Autodesk Inventor part; units mm, degrees
ref_plane "YZ Plane" through (0, 0, 0) normal (1, 0, 0) x (0, 1, 0)
ref_plane "XZ Plane" through (0, 0, 0) normal (0, 1, 0) x (-1, 0, 0)
ref_plane "XY Plane" through (0, 0, 0) normal (0, 0, 1) x (1, 0, 0)
sketch "Sketch1" plane through (0, 0, 0) normal (1, 0, 0) x (0, 1, 0)
  line L0 (-50, 45) -> (50, 45)
  line L1 (50, 45) -> (50, -45)
  line L2 (50, -45) -> (-50, -45)
  line L3 (-50, -45) -> (-50, 45)
  point P0 (0, 0)
  dimension "d0" = 100
  dimension "d35" = 90
  dimension "d36" = 50
  dimension "d37" = 45
extrude "Plate1" add sketch "Sketch1" along normal blind 3
sketch "Sketch2" plane through (-3, 53, -45) normal (0, 1, 0) x (-1, 0, 0)
  line L0 (0, 90) -> (0, 0)
  line L1 (0, 0) -> (19, 0)
  line L2 (19, 0) -> (19, 90)
  line L3 (19, 90) -> (0, 90)
edge flange "Flange1" height 25 angle 90 thickness 3 bend radius 3 thickness toward (0, 1, 0) relief tear relief width 3 relief depth 1.5 corner gap 3 corner form 0 edges at (0, 50, 0) (0, -50, 0) wall of the first edge with corners at (-3, 53, 45) (-3, 53, -45) (-22, 53, -45) (-22, 53, 45)
bend "Bend1"
corner "Corner1"
sketch "Sketch3" plane through (6, -50, 48) normal (0, 0, 1) x (1, 0, 0)
  line L0 (0, 100) -> (0, 0)
  line L1 (0, 0) -> (23.4696, 0)
  line L2 (23.4696, 0) -> (23.4696, 100)
  line L3 (23.4696, 100) -> (0, 100)
edge flange "Flange2" height 29.4696 angle 90 thickness 3 bend radius 3 thickness toward (0, 0, 1) relief tear relief width 3 relief depth 1.5 corner gap 3 corner form 0 edges at (3, 0, 45) (3, 0, -45) wall of the first edge with corners at (6, 50, 48) (6, -50, 48) (29.4696, -50, 48) (29.4696, 50, 48)
bend "Bend2"
corner "Corner2"
sketch "Sketch4" plane through (3, 0, 0) normal (1, 0, 0) x (0, 0, -1)
  line L0 (-45, 50) -> (45, 50)
  line L1 (-45, -50) -> (-45, 50)
  line L2 (45, -50) -> (-45, -50)
  line L3 (45, 50) -> (45, -50)
  circle A0 centre (-31.5962, 12.4637) radius 7.62 construction
  circle A1 centre (1.5, 12.4637) radius 12.7 construction
  circle A2 centre (34.5962, 12.4637) radius 7.62 construction
  circle A3 centre (1.5, -25.7125) radius 25.4 construction
  circle A4 centre (1.5, 12.4637) radius 25.4 construction
  line L4 (26.9762, 12.4637) -> (26.9, 12.4637) construction
  line L5 (-23.9762, 12.4637) -> (-23.9, 12.4637) construction
  line L6 (1.5, -0.3125) -> (1.5, -0.2363) construction
  line L7 (-33.5, -12.8649) -> (-29.6924, 37.7923) construction
  line L8 (36.5, -12.8649) -> (32.6924, 37.7923) construction
  point P0 (0, 0)
  dimension "d24" = 25.4
  dimension "d25" = 15.24
  dimension "d27" = 50.8
  dimension "d23" = 0.0762
  dimension "d26" = 50.8
  dimension "d34" = 66.1924
  dimension "d38" = 24.2875
  dimension "d40" = 46.5
  dimension "d41" = 43.5
  dimension "d42" = 50.8
  dimension "d45" = 70
sketch "Sketch5" plane through (3, 0, 0) normal (1, 0, 0) x (0, 0, -1)
  circle A0 centre (-31.5962, 12.4637) radius 9.525
  circle A1 centre (34.5962, 12.4637) radius 9.525
  circle A2 centre (1.5, 12.4637) radius 11.1125
  circle A3 centre (1.5, -25.7125) radius 14.2875
  line L0 (-33.5, -12.8649) -> (-29.6924, 37.7923) construction
  line L1 (36.5, -12.8649) -> (32.6924, 37.7923) construction
  circle A4 centre (-29.6924, 37.7923) radius 3
  circle A5 centre (32.6924, 37.7923) radius 3
  circle A6 centre (36.5, -12.8649) radius 3
  circle A7 centre (-33.5, -12.8649) radius 3
  point P0 (0, 0)
  dimension "d28" = 19.05
  dimension "d30" = 22.225
  dimension "d31" = 28.575
  dimension "d44" = 6
extrude "Cut1" cut sketch "Sketch5" against normal blind 3
sketch "Sketch7" plane through (29.4696, -50, 51) normal (0, 0, 1) x (1, 0, 0)
  line L0 (-23.4696, 100) -> (-23.4696, 0)
  line L1 (0, 100) -> (0, 0)
  line L2 (-23.4696, 100) -> (0, 100)
  circle A0 centre (-11.7348, 90) radius 3
  circle A1 centre (-11.7348, 55) radius 3
  circle A2 centre (-11.7348, 20) radius 3
  point P0 (-29.4696, 50)
  dimension "d72" = 6
  dimension "d74" = 11.7348
  dimension "d75" = 11.7348
  dimension "d76" = 10
  dimension "d79" = 35
extrude "Cut3" cut sketch "Sketch7" against normal through all
sketch "Sketch8" plane through (-22, 56, 45) normal (0, 1, 0) x (1, 0, 0)
  line L0 (19, 0) -> (19, 90)
  line L1 (0, 0) -> (0, 90)
  line L2 (19, 0) -> (0, 0)
  circle A0 centre (9.5, 15) radius 3
  circle A1 centre (9.5, 35) radius 3
  circle A2 centre (9.5, 55) radius 3
  circle A3 centre (9.5, 75) radius 3
  point P0 (22, 45)
  dimension "d86" = 6
  dimension "d88" = 9.5
  dimension "d89" = 9.5
  dimension "d90" = 15
  dimension "d93" = 20
extrude "Cut4" cut sketch "Sketch8" against normal through all
sketch "Sketch9" plane through (0, 0, 0) normal (-1, 0, 0) x (0, 0, 1)
  circle A0 centre (-1.5, 12.4637) radius 11.1125
  circle A1 centre (-32.6924, 37.7923) radius 3
  circle A2 centre (-34.5962, 12.4637) radius 9.525
  line L0 (45, 50) -> (-45, 50)
  arc A3 (-20.715, 19.4163) -> (-27.9683, 26.5028) centre (-34.5962, 12.4637) ccw
  arc A4 (-28.1286, 30.0352) -> (-24.3769, 41.235) centre (-32.6924, 37.7923) ccw
  arc A5 (-5.9768, 28.9802) -> (-17.1032, 19.4907) centre (-1.5, 12.4637) ccw
  line L1 (-6.5, 44) -> (-22.529, 44)
  arc A6 (-28.1286, 30.0352) -> (-27.9683, 26.5028) centre (-27.1145, 28.3114) ccw
  arc A7 (-22.529, 44) -> (-24.3769, 41.235) centre (-22.529, 42) ccw
  arc A8 (-20.715, 19.4163) -> (-17.1032, 19.4907) centre (-18.9268, 20.3119) ccw
  circle A9 centre (-36.5, -12.8649) radius 3
  circle A10 centre (-1.5, -25.7125) radius 14.2875
  line L2 (-45, 50) -> (-45, -50)
  line L3 (-45, -50) -> (45, -50)
  line L4 (-4.5, 30.9106) -> (-4.5, 42)
  arc A11 (-4.5, 42) -> (-6.5, 44) centre (-6.5, 42) ccw
  arc A12 (-5.9768, 28.9802) -> (-4.5, 30.9106) centre (-6.5, 30.9106) ccw
  line L5 (-1.5, 12.4637) -> (-1.5, -25.7125)
  arc A13 (-21.6278, -23.1723) -> (-15.3483, -40.5384) centre (-1.5, -25.7125) ccw
  arc A14 (-36.9091, -21.8555) -> (-30.3842, -19.4676) centre (-36.5, -12.8649) ccw
  line L6 (-39, -23.8535) -> (-39, -42)
  line L7 (-16.7135, -44) -> (-37, -44)
  arc A15 (-39, -42) -> (-37, -44) centre (-37, -42) ccw
  arc A16 (-16.7135, -44) -> (-15.3483, -40.5384) centre (-16.7135, -42) ccw
  arc A17 (-36.9091, -21.8555) -> (-39, -23.8535) centre (-37, -23.8535) ccw
  line L8 (-28.3359, -19.0574) -> (-22.9229, -21.0444)
  arc A18 (-28.3359, -19.0574) -> (-30.3842, -19.4676) centre (-29.0251, -20.9349) ccw
  arc A19 (-21.6278, -23.1723) -> (-22.9229, -21.0444) centre (-23.6121, -22.9219) ccw
  arc A20 (-27.5648, -11.7869) -> (-30.828, -5.8772) centre (-36.5, -12.8649) ccw
  arc A21 (-8.7645, -6.7702) -> (-18.4911, -14.6272) centre (-1.5, -25.7125) ccw
  arc A22 (-17.1032, 5.4367) -> (-8.6455, -3.0855) centre (-1.5, 12.4637) ccw
  arc A23 (-30.1414, -2.4084) -> (-20.715, 5.5111) centre (-34.5962, 12.4637) ccw
  line L9 (-26.2684, -13.4249) -> (-20.8554, -15.4119)
  arc A24 (-27.5648, -11.7869) -> (-26.2684, -13.4249) centre (-25.5792, -11.5474) ccw
  arc A25 (-30.1414, -2.4084) -> (-30.828, -5.8772) centre (-29.5675, -4.3243) ccw
  arc A26 (-17.1032, 5.4367) -> (-20.715, 5.5111) centre (-18.9268, 4.6155) ccw
  arc A27 (-8.7645, -6.7702) -> (-8.6455, -3.0855) centre (-9.4807, -4.9028) ccw
  arc A28 (-20.8554, -15.4119) -> (-18.4911, -14.6272) centre (-20.1662, -13.5344) ccw
  arc A29 (24.9683, 26.5028) -> (17.715, 19.4163) centre (31.5962, 12.4637) ccw
  arc A30 (21.3769, 41.235) -> (25.1286, 30.0352) centre (29.6924, 37.7923) ccw
  arc A31 (14.1032, 19.4907) -> (2.9768, 28.9802) centre (-1.5, 12.4637) ccw
  line L10 (3.5, 44) -> (19.529, 44)
  arc A32 (24.9683, 26.5028) -> (25.1286, 30.0352) centre (24.1145, 28.3114) ccw
  arc A33 (21.3769, 41.235) -> (19.529, 44) centre (19.529, 42) ccw
  arc A34 (14.1032, 19.4907) -> (17.715, 19.4163) centre (15.9268, 20.3119) ccw
  line L11 (1.5, 30.9106) -> (1.5, 42)
  arc A35 (3.5, 44) -> (1.5, 42) centre (3.5, 42) ccw
  arc A36 (1.5, 30.9106) -> (2.9768, 28.9802) centre (3.5, 30.9106) ccw
  arc A37 (12.3483, -40.5384) -> (18.6278, -23.1723) centre (-1.5, -25.7125) ccw
  arc A38 (27.3842, -19.4676) -> (33.9091, -21.8555) centre (33.5, -12.8649) ccw
  line L12 (36, -23.8535) -> (36, -42)
  line L13 (13.7135, -44) -> (34, -44)
  arc A39 (34, -44) -> (36, -42) centre (34, -42) ccw
  arc A40 (12.3483, -40.5384) -> (13.7135, -44) centre (13.7135, -42) ccw
  arc A41 (36, -23.8535) -> (33.9091, -21.8555) centre (34, -23.8535) ccw
  line L14 (25.3359, -19.0574) -> (19.9229, -21.0444)
  arc A42 (27.3842, -19.4676) -> (25.3359, -19.0574) centre (26.0251, -20.9349) ccw
  arc A43 (19.9229, -21.0444) -> (18.6278, -23.1723) centre (20.6121, -22.9219) ccw
  arc A44 (27.828, -5.8772) -> (24.5648, -11.7869) centre (33.5, -12.8649) ccw
  arc A45 (15.4911, -14.6272) -> (5.7645, -6.7702) centre (-1.5, -25.7125) ccw
  arc A46 (5.6455, -3.0855) -> (14.1032, 5.4367) centre (-1.5, 12.4637) ccw
  arc A47 (17.715, 5.5111) -> (27.1414, -2.4084) centre (31.5962, 12.4637) ccw
  line L15 (23.2684, -13.4249) -> (17.8554, -15.4119)
  arc A48 (23.2684, -13.4249) -> (24.5648, -11.7869) centre (22.5792, -11.5474) ccw
  arc A49 (27.828, -5.8772) -> (27.1414, -2.4084) centre (26.5675, -4.3243) ccw
  arc A50 (17.715, 5.5111) -> (14.1032, 5.4367) centre (15.9268, 4.6155) ccw
  arc A51 (5.6455, -3.0855) -> (5.7645, -6.7702) centre (6.4807, -4.9028) ccw
  arc A52 (15.4911, -14.6272) -> (17.8554, -15.4119) centre (17.1662, -13.5344) ccw
  point P0 (0, 0)
  point P1 (-26.176, 44)
  dimension "d100" = 6
  dimension "d101" = 6
  dimension "d102" = 6
  dimension "d103" = 6
  dimension "d105" = 2
  dimension "d108" = 6
  dimension "d109" = 6
  dimension "d110" = 3
  dimension "d111" = 6
  dimension "d112" = 6
  dimension "d113" = 3
  dimension "d114" = 6
cut "Cut5" [suppressed]
equation "\"d32\" = Thickness"
equation "\"d3\" = BendReliefWidth"
equation "\"d4\" = BendReliefDepth"
equation "\"d5\" = MinimumRemnant"
equation "\"d6\" = BendRadius"
equation "\"d9\" = BendRadius"
equation "\"d10\" = CornerReliefSize"
equation "\"d11\" = GapSize"
equation "\"d12\" = JacobiRadiusSize"
equation "\"d13\" = BendReliefWidth"
equation "\"d14\" = BendReliefDepth"
equation "\"d15\" = MinimumRemnant"
equation "\"d16\" = BendRadius"
equation "\"d19\" = BendRadius"
equation "\"d20\" = CornerReliefSize"
equation "\"d21\" = GapSize"
equation "\"d22\" = JacobiRadiusSize"
equation "\"BendRadius\" = Thickness"
equation "\"BendReliefWidth\" = Thickness"
equation "\"BendReliefDepth\" = 0.5 * Thickness"
equation "\"CornerReliefSize\" = 4 * Thickness"
equation "\"MinimumRemnant\" = 2 * Thickness"
equation "\"TransitionRadius\" = BendRadius"
equation "\"JacobiRadiusSize\" = BendRadius"
equation "\"GapSize\" = Thickness"
equation "\"d2\" = BendRadius"
properties part number "GearboxPlate" material "Aluminum 6061"
Part model, mm, in its own coordinate system. A direction names the side the tool comes from. Round coordinates to 2 decimals unless told otherwise and drop trailing zeros. Write each loop counter-clockwise with the first axis right and the second up, starting at its lowest first coordinate (ties: lowest second). Pieces come first, ordered by that corner, then holes. Notation, with made-up numbers: (3, 85.25) -> (8, 85.25) arc R27 cw to (8, 113.25) -> close; hole circle Ø7 at (64, 50). An arc over 180 degrees is marked (long way). Return JSON: item names as keys, results as strings. Group by question number.
Q1. Probe L1, parallel to Y at x = -14.5, z = 15.5; L2, parallel to Y at x = 1, z = -36; L3, parallel to Z at x = 19, y = -1. List the from-to ranges inside material, lowest first. Write a range as [from, to].
Q2. Which spindle directions (+Z, -Z, +X, -X, +Y, -Y) get a long thin tool onto all of the face, cutting with end or side? Do faces 1 (the flat face through (-10, 54, 45)), 2 (the flat face through (18, 1, -48)), 3 (the cylindrical face through (-0.9, -52.14, 0.63)). Say none if no direction does.
Q3. Saw through at D-D on x = 7.5. Write the cut outline in (y, z).
Q4. Saw through at B-B on z = -1.5. Write the cut outline in (x, y) (3 decimals), plus the area to 3 significant figures.
Q5. Pin check, flat tips, straight feed: pin 1 (6 mm diameter, centred on x = -4.5, y = -19, fed in from -Z); pin 2 (2 mm diameter, centred on y = -37.5, z = -11, fed in from +X); pin 3 (3 mm diameter, centred on y = -2, z = -7, fed in from -X); pin 4 (5 mm diameter, centred on x = 0, y = 22, fed in from +Z). Stop position of each tip, or through.
Q6. Saw through at C-C on y = 18. Write the cut outline in (x, z), plus the area to 3 significant figures.
Q7. Saw through at A-A on x = -7.5. Write the cut outline in (y, z), plus the area to 3 significant figures.
Q8. Mould opens along X. For faces 4 (the flat face through (0, -1, 1)), 5 (the flat face through (15, -50, -49)), 6 (the cylindrical face through (-14.71, -54.48, -32.03)), 7 (the cylindrical face through (-14.71, -54.48, 7.97)) say: pulls with the +X half, pulls with the -X half, needs draft (parallel to the pull), parting line crosses it, or undercut.
Answer:
{
 "1": {"L1": "[-56, -53], [53, 56]", "L2": "[-54.47, -15.82], [-9.91, 3.04], [21.88, 54.47]", "L3": "[-51, -48], [48, 51]"},
 "2": {"face 1": "+Z, +X, -X, +Y", "face 2": "+X, +Y, -Y", "face 3": "+Z, -Z, -X"},
 "3": {"outline": "(-50, -51) -> (50, -51) -> (50, -48) -> (-50, -48) -> close; (-50, 48) -> (50, 48) -> (50, 51) -> (-50, 51) -> close"},
 "4": {"outline": "(-22, -56) -> (-3, -56) arc R6 ccw to (3, -50) -> (3, -40) -> (0, -40) -> (0, -50) arc R3 cw to (-3, -53) -> (-22, -53) -> close; (-22, 53) -> (-3, 53) arc R3 cw to (0, 50) -> (0, 23.576) -> (3, 23.576) -> (3, 50) arc R6 ccw to (-3, 56) -> (-22, 56) -> close; (0, -11.425) -> (3, -11.425) -> (3, 1.351) -> (0, 1.351) -> close", "area": "304 mm2"},
 "5": {"pin 1": "through", "pin 2": "x = 3", "pin 3": "x = 0", "pin 4": "z = 49.87"},
 "6": {"outline": "(0, -45) arc R6 ccw to (6, -51) -> (29.47, -51) -> (29.47, -48) -> (6, -48) arc R3 cw to (3, -45) -> (3, -42.35) -> (0, -42.35) -> close; (0, -26.85) -> (3, -26.85) -> (3, -11.14) -> (0, -11.14) -> close; (0, 8.14) -> (3, 8.14) -> (3, 23.85) -> (0, 23.85) -> close; (0, 39.35) -> (3, 39.35) -> (3, 45) arc R3 cw to (6, 48) -> (29.47, 48) -> (29.47, 51) -> (6, 51) arc R6 ccw to (0, 45) -> close", "area": "302 mm2"},
 "7": {"outline": "(-56, -45) -> (-53, -45) -> (-53, 45) -> (-56, 45) -> close; (53, -45) -> (56, -45) -> (56, 45) -> (53, 45) -> close", "area": "540 mm2"},
 "8": {"face 4": "pulls with the -X half", "face 5": "needs draft", "face 6": "undercut", "face 7": "undercut"}
}
